Input: dimensioned drawing with shaded views. Units: mm. Origin: part minimum x, y, z. A direction names the side the tool comes from. Give positions to 0.01 mm unless a question says otherwise; leave off trailing zeros. Loops run counter-clockwise (first coordinate to the right, second up) from the corner with the lowest first, then second, coordinate; pieces in that order, holes last. Notation, with made-up numbers: (70.25, 28.5) -> (97.25, 28.5) arc R35 cw to (97.25, 67.5) -> close; hole circle Ø7 at (18.25, -17.75). An arc over 180 degrees is marked (long way). Answer in a Markdown table with one row per item. Add a question column.
1) First-contact query: P1, Ø4, axis at y = 1.5, z = 7.5, coming from the -X side; P2, Ø2, axis at y = 4.5, z = 9.5, coming from the +X side; P3, Ø2.5, axis at x = 6.5, z = 7, coming from the -Y side. Flat tips, straight axial feed; report the tip coordinate or a pass-through.
2) Access query for the marked faces 4 and 5. Directions: +Z, -Z, +X, -X, +Y, -Y. A direction counts if a zero-diameter tool reaches every point of the face in a straight line with its end or side. Return the directions, or none.
3) Section query B-B (z = 8). Return the cut outline in (x, y).
4) Section query C-C (x = 6.5). Return the cut outline in (y, z), plus the area to 3 significant figures.
5) Draft query along Z for the marked faces 1, 2 and 3. Return one class per face: +Z half, -Z half, draft (parallel to the pull), parting line (faces both ways), or undercut.
6) Line query: line 1 (Y direction, x = 8.25, z = 5.25); line 2 (Z direction, x = 6.5, y = 2.4); line 3 (Y direction, x = 3.75, z = 5.25). Output: solid intervals per line, ascending. Write a range as from..to.
7) Section query D-D (y = 2). Return the cut outline in (x, z).
8) Section query A-A (z = 6.5). Return the cut outline in (x, y), plus the area to 3 significant figures.
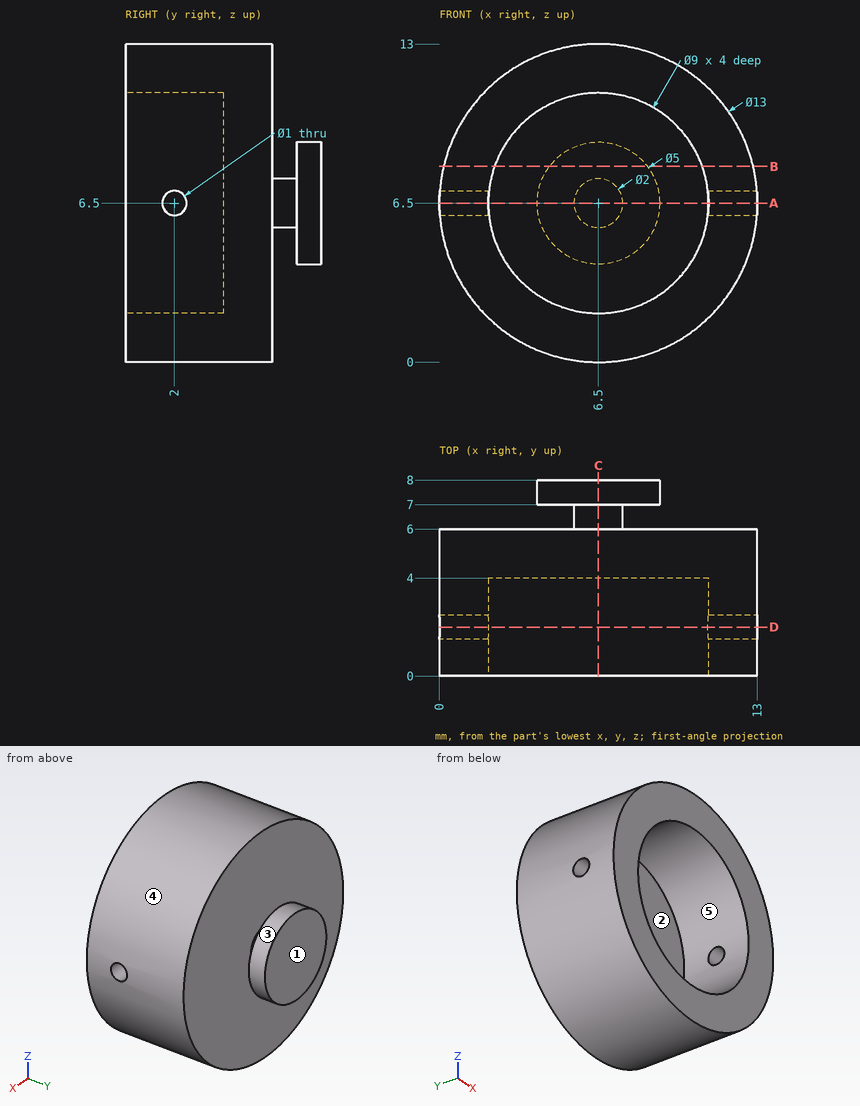
Evaluation:
| question | item | result |
|---|---|---|
| 1 | P1 | x = 0 |
| 1 | P2 | x = 12.68 |
| 1 | P3 | y = 4 |
| 2 | face 4 | +Y, -Y |
| 2 | face 5 | -Y |
| 3 | outline | (0.18, 0) -> (2.26, 0) -> (2.26, 4) -> (10.74, 4) -> (10.74, 0) -> (12.82, 0) -> (12.82, 6) -> (0.18, 6) -> close; (4.5, 7) -> (8.5, 7) -> (8.5, 8) -> (4.5, 8) -> close |
| 4 | outline | (0, 0) -> (6, 0) -> (6, 5.5) -> (7, 5.5) -> (7, 4) -> (8, 4) -> (8, 9) -> (7, 9) -> (7, 7.5) -> (6, 7.5) -> (6, 13) -> (0, 13) -> (0, 11) -> (4, 11) -> (4, 2) -> (0, 2) -> close |
| 4 | area | 49.0 mm² |
| 5 | face 1 | draft |
| 5 | face 2 | undercut |
| 5 | face 3 | parting line |
| 6 | line 1 | 4..6, 7..8 |
| 6 | line 2 | 0..2, 11..13 |
| 6 | line 3 | 4..6 |
| 7 | outline | (0.02, 6) arc R6.5 ccw to (12.98, 6) -> (10.97, 6) arc R4.5 cw to (2.03, 6) -> close; (0.02, 7) -> (2.03, 7) arc R4.5 cw to (10.97, 7) -> (12.98, 7) arc R6.5 ccw to start |
| 8 | outline | (0, 0) -> (2, 0) -> (2, 1.5) -> (0, 1.5) -> close; (0, 2.5) -> (2, 2.5) -> (2, 4) -> (11, 4) -> (11, 2.5) -> (13, 2.5) -> (13, 6) -> (7.5, 6) -> (7.5, 7) -> (9, 7) -> (9, 8) -> (4, 8) -> (4, 7) -> (5.5, 7) -> (5.5, 6) -> (0, 6) -> close; (11, 0) -> (13, 0) -> (13, 1.5) -> (11, 1.5) -> close |
| 8 | area | 45.0 mm² |
